Check sheet for the modelled part. Datum: model origin and axes. Units: mm. Give positions to 0.01 mm unless a question says otherwise; leave off trailing zeros. Order: outer loops, then holes, each group sorted by start corner. A loop starts at its lowest first (then second) coordinate and runs counter-clockwise, first axis right, second up.
Item 1: Sectioned sample at B-B on z = 2.95. Record the boundary of the cut face in (x, y).
Item 2: Sectioned sample at A-A on y = -17.5. Record the boundary of the cut face in (x, z).
Item 3: Gauge pin test, flat ends, axial feed: P1, Ø3, axis at x = 238.85, y = -82.29, coming from the -Z side; P2, Ø0.6, axis at x = 147.5, z = 2.5, coming from the +Y side. Record the tip position at first contact, or that the pin passes through.
Item 4: Sectioned sample at D-D on x = 87. Record the boundary of the cut face in (y, z).
Item 5: Material ranges on line 1 along Y through (x, z) = (143.5, 3.3); line 2 along X through (y, z) = (-28, 3.25); line 3 along Y through (x, z) = (156.5, 3.1), recorded low to high.
Item 6: Sectioned sample at C-C on x = 44. Record the boundary of the cut face in (y, z).
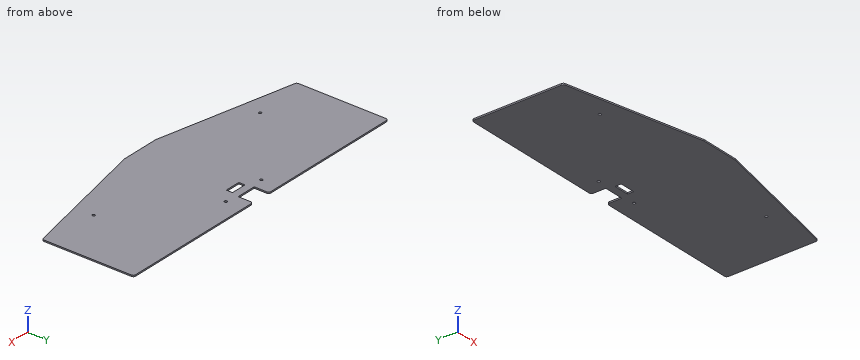
from build123d import *

# Parameters (mm, degrees)
SKETCH006_W     = 13.6
SKETCH006_H     = 5.5
PAD001_DEPTH    = 1.2
FILLET001_R     = 2
SKETCH011_R     = 1.2
POCKET001_DEPTH = 1.2


with BuildPart() as part:
    # Sketch006 (on DatumPlane) → Pad001 (new body)
    with BuildSketch(Plane.XY.offset(2.2)):
        Polygon((9.202145, -8.293724), (9.202145, -88.808503), (130.974502, -114.692017), (165.022509, -114.692017), (286.852356, -88.796284), (286.852356, -8.293724), (156.82725, -8.293724), (156.82725, -21.293724), (139.22725, -21.293724), (139.22725, -8.293724), align=None)
        with Locations((148.02725, -30.543724)):
            Rectangle(SKETCH006_W, SKETCH006_H, mode=Mode.SUBTRACT)
    extrude(amount=PAD001_DEPTH)

    # Fillet001
    fillet001_edges = [part.edges().sort_by_distance(p)[0] for p in [
        (9.202145, -8.293724, 2.8),
        (9.202145, -88.808503, 2.8),
        (156.82725, -8.293724, 2.8),
        (139.22725, -8.293724, 2.8),
        (286.852356, -8.293724, 2.8),
        (130.974502, -114.692017, 2.8),
        (165.022509, -114.692017, 2.8),
        (286.852356, -88.796284, 2.8),
    ]]
    fillet(fillet001_edges, radius=FILLET001_R)

    # Sketch011 (on Face5 of Fillet001) → Pocket001 (cut)
    with BuildSketch(Plane.XY.offset(3.4)):
        with Locations((128.72725, -23.589033)):
            Circle(SKETCH011_R)
        with Locations((167.327251, -23.589033)):
            Circle(SKETCH011_R)
        with Locations((238.852356, -82.293724)):
            Circle(SKETCH011_R)
        with Locations((57.202145, -82.293724)):
            Circle(SKETCH011_R)
    extrude(amount=-POCKET001_DEPTH, mode=Mode.SUBTRACT)


solid = part.part
Report:
1. outline: (9.2, -87.19) arc R2 ccw to (10.79, -89.15) - (130.77, -114.65) arc R2 ccw to (131.18, -114.69) - (164.81, -114.69) arc R2 ccw to (165.23, -114.65) - (285.27, -89.13) arc R2 ccw to (286.85, -87.18) - (286.85, -10.29) arc R2 ccw to (284.85, -8.29) - (158.83, -8.29) arc R2 ccw to (156.83, -10.29) - (156.83, -21.29) - (139.23, -21.29) - (139.23, -10.29) arc R2 ccw to (137.23, -8.29) - (11.2, -8.29) arc R2 ccw to (9.2, -10.29) - close; hole circle Ø2.4 at (57.2, -82.29); hole circle Ø2.4 at (128.73, -23.59); hole (141.23, -33.29) - (154.83, -33.29) - (154.83, -27.79) - (141.23, -27.79) - close; hole circle Ø2.4 at (167.33, -23.59); hole circle Ø2.4 at (238.85, -82.29)
2. outline: (9.2, 2.2) - (139.23, 2.2) - (139.23, 3.4) - (9.2, 3.4) - close; (156.83, 2.2) - (286.85, 2.2) - (286.85, 3.4) - (156.83, 3.4) - close
3. P1: stops at z = 2.2
3. P2: stops at y = -21.29
4. outline: (-105.34, 2.2) - (-8.29, 2.2) - (-8.29, 3.4) - (-105.34, 3.4) - close
5. line 1: y = -114.69 to -33.29, -27.79 to -21.29
5. line 2: x = 9.2 to 141.23, 154.83 to 286.85
5. line 3: y = -114.69 to -21.29
6. outline: (-96.21, 2.2) - (-8.29, 2.2) - (-8.29, 3.4) - (-96.21, 3.4) - close
